Geometry check sheet. Reference: the model listing, model coordinates, mm. A direction names the side the tool comes from. Round coordinates to 2 decimals unless told otherwise and drop trailing zeros. Order: outer loops, then holes, each group sorted by start corner. A loop starts at its lowest first (then second) coordinate and runs counter-clockwise, first axis right, second up.
(1) Cross-section at B-B on x = 0. Enter the section's corners in (y, z).
(2) Draft check along Y on faces 1 (the face through (13, -6, -1)), 2 (the face through (7.483, -6.069, -0.784)), 3 (the face through (9, -15, -1)), 4 (the face through (-9, 15, -1)). Enter one of: pulls with the +Y half, pulls with the -Y half, needs draft (parallel to the pull), parting line crosses it, or undercut.
(3) Set-up check for faces 5 (the face through (-5, -2, -56)), 6 (the face through (6, 13, -1)): record each of +Z, -Z, +X, -X, +Y, -Y from which the full face is reachable in a straight line by a thin tool's end or side.
(4) Cross-section at A-A on y = 11.25. Enter the section's corners in (x, z), and give its area (3 significant figures).
(5) Thickness scan on L1, parallel to Y at x = 10.25, z = -46.5; L2, parallel to Y at x = 0, z = 0.5. Record the ranges inside material, lowest first.
(6) Gauge pin test, flat ends, axial feed: P1, Ø3, axis at y = -3, z = 41.5, coming from the -X side; P2, Ø0.8, axis at x = 4.5, z = 27.5, coming from the -Y side; P3, Ø0.8, axis at x = -4.5, z = -4, coming from the +Y side. Record the tip position at first contact, or that the pin passes through.
Autodesk Inventor part; units mm, degrees
ref_plane "YZ Plane" through (0, 0, 0) normal (1, 0, 0) x (0, 1, 0)
ref_plane "XZ Plane" through (0, 0, 0) normal (0, 1, 0) x (-1, 0, 0)
ref_plane "XY Plane" through (0, 0, 0) normal (0, 0, 1) x (1, 0, 0)
sketch "Sketch1" plane through (0, 0, 0) normal (0, 0, 1) x (1, 0, 0)
  circle A0 centre (0, 0) radius 5
  arc A1 (-13, 15) -> (-15, 13) centre (-13, 13) ccw
  arc A2 (-15, -13) -> (-13, -15) centre (-13, -13) ccw
  arc A3 (13, -15) -> (15, -13) centre (13, -13) ccw
  arc A4 (15, 13) -> (13, 15) centre (13, 13) ccw
  arc A5 (-13, 14) -> (-14, 13) centre (-13, 13) ccw
  arc A6 (-14, -13) -> (-13, -14) centre (-13, -13) ccw
  arc A7 (13, -14) -> (14, -13) centre (13, -13) ccw
  arc A8 (14, 13) -> (13, 14) centre (13, 13) ccw
  line L0 (14, -14) -> (-14, 14) construction
  line L1 (-14, -14) -> (14, 14) construction
  line L2 (15, -15) -> (-15, 15) construction
  line L3 (-15, -15) -> (15, 15) construction
  line L4 (-13, 15) -> (-8, 15)
  line L5 (-8, 13) -> (-8, 8) construction
  line L6 (-9.4142, 8) -> (-13, 8)
  line L7 (-15, 8) -> (-15, 13)
  line L8 (-13, -15) -> (-8, -15)
  line L9 (-8, -13) -> (-8, -9.4142)
  line L10 (-9.4142, -8) -> (-13, -8)
  line L11 (-15, -8) -> (-15, -13)
  line L12 (13, -15) -> (8, -15)
  line L13 (8, -13) -> (8, -9.4142)
  line L14 (9.4142, -8) -> (13, -8)
  line L15 (15, -8) -> (15, -13)
  line L16 (13, 15) -> (8, 15)
  line L17 (8, 13) -> (8, 9.4142)
  line L18 (9.4142, 8) -> (13, 8)
  line L19 (15, 8) -> (15, 13)
  line L20 (-13, 9) -> (-10, 9)
  line L21 (-9, 10) -> (-9, 13)
  line L22 (-10, 14) -> (-13, 14)
  line L23 (-14, 13) -> (-14, 10)
  line L24 (13, 9) -> (10, 9)
  line L25 (9, 10) -> (9, 13)
  line L26 (10, 14) -> (13, 14)
  line L27 (14, 13) -> (14, 10)
  line L28 (13, -9) -> (10, -9)
  line L29 (9, -10) -> (9, -13)
  line L30 (10, -14) -> (13, -14)
  line L31 (14, -13) -> (14, -10)
  line L32 (-13, -9) -> (-10, -9)
  line L33 (-9, -10) -> (-9, -13)
  line L34 (-10, -14) -> (-13, -14)
  line L35 (-14, -13) -> (-14, -10)
  line L36 (-14, 13) -> (-14, 10)
  line L37 (-14, -10) -> (-14, -13)
  line L38 (-14, -13) -> (-14, -10)
  line L39 (-14, 10) -> (-14, 13)
  line L40 (13, -15) -> (5, -15)
  line L41 (-5, -15) -> (-13, -15)
  line L42 (13, -15) -> (5, -15) construction
  line L43 (0, -15) -> (-13, -15) construction
  line L44 (4, -13) -> (8, -13)
  line L45 (-8, -13) -> (-4, -13)
  line L46 (10, -9) -> (13, -9)
  line L47 (14, -10) -> (14, -13)
  line L48 (13, -14) -> (10, -14)
  line L49 (9, -13) -> (9, -10)
  line L50 (5, -14) -> (5, -15)
  line L51 (13, -14) -> (10, -14)
  line L52 (5, -14) -> (4, -14)
  line L53 (4, -14) -> (5, -14)
  line L54 (10, -14) -> (13, -14)
  line L55 (-4, -14) -> (-5, -14)
  line L56 (-10, -14) -> (-13, -14)
  line L57 (-13, -14) -> (-10, -14)
  line L58 (-5, -14) -> (-4, -14)
  line L59 (14, -13) -> (14, -10)
  line L60 (14, 10) -> (14, 13)
  line L61 (14, 13) -> (14, 10)
  line L62 (14, -10) -> (14, -13)
  line L63 (-5, -14) -> (-5, -15)
  line L64 (10, 14) -> (13, 14)
  line L65 (13, 14) -> (10, 14)
  line L66 (-10, 14) -> (-13, 14)
  line L67 (-13, 14) -> (-10, 14)
  line L68 (-5, 15) -> (-5, 14)
  line L69 (-13, 15) -> (-5, 15)
  line L70 (5, 15) -> (13, 15)
  line L71 (-15, 15) -> (-5, 15) construction
  line L72 (5, 15) -> (15, 15) construction
  line L73 (5, 15) -> (5, 14)
  line L74 (8, 13) -> (4, 13)
  line L75 (5, 14) -> (4, 14)
  line L76 (-5, 14) -> (-4, 14)
  line L77 (4, 14) -> (5, 14)
  line L78 (-4, 13) -> (-8, 13)
  line L79 (-4, 14) -> (-5, 14)
  line L80 (4, 13) -> (4, 14)
  line L81 (-4, 13) -> (-4, 14)
  line L82 (-4, -14) -> (-4, -13)
  line L83 (4, -14) -> (4, -13)
  line L84 (-8, 9.4142) -> (-4.1919, 5.6061)
  line L85 (8, 9.4142) -> (4.1919, 5.6061)
  line L86 (9.4142, 8) -> (5.6061, 4.1919)
  line L87 (5.6061, -4.1919) -> (9.4142, -8)
  line L88 (4.1919, -5.6061) -> (8, -9.4142)
  line L89 (-4.1919, -5.6061) -> (-8, -9.4142)
  line L90 (-5.6061, -4.1919) -> (-9.4142, -8)
  line L91 (-9.4142, 8) -> (-5.6061, 4.1919)
  arc A9 (4.1919, 5.6061) -> (-4.1919, 5.6061) centre (0, 0) ccw
  arc A10 (5.6061, -4.1919) -> (5.6061, 4.1919) centre (0, 0) ccw
  arc A11 (-5.6061, 4.1919) -> (-5.6061, -4.1919) centre (0, 0) ccw
  arc A12 (-4.1919, -5.6061) -> (4.1919, -5.6061) centre (0, 0) ccw
  line L92 (-8, 13) -> (-8, 9.4142)
  line L93 (-15, -13) -> (-15, -5) construction
  line L94 (-15, -13) -> (-15, -5)
  line L95 (-15, 5) -> (-15, 13)
  line L96 (15, -5) -> (15, -13) construction
  line L97 (15, 13) -> (15, 5)
  line L98 (15, -5) -> (15, -13)
  line L99 (-14, -4) -> (-14, -5)
  line L100 (14, -4) -> (14, -5)
  line L101 (14, 4) -> (14, 5)
  line L102 (-14, 4) -> (-14, 5)
  line L103 (-13, 8) -> (-13, 4)
  line L104 (13, 4) -> (13, 8)
  line L105 (13, -8) -> (13, -4)
  line L106 (-13, -4) -> (-13, -8)
  line L107 (-14, -5) -> (-15, -5)
  line L108 (15, -5) -> (14, -5)
  line L109 (15, 5) -> (14, 5)
  line L110 (-14, 5) -> (-15, 5)
  line L111 (13, 4) -> (14, 4)
  line L112 (-14, 4) -> (-13, 4)
  line L113 (-14, -4) -> (-13, -4)
  line L114 (13, -4) -> (14, -4)
  arc A13 (-13, -9) -> (-14, -10) centre (-13, -10) ccw
  arc A14 (-9, -10) -> (-10, -9) centre (-10, -10) ccw
  arc A15 (-10, -14) -> (-9, -13) centre (-10, -13) ccw
  arc A16 (10, -9) -> (9, -10) centre (10, -10) ccw
  arc A17 (9, -13) -> (10, -14) centre (10, -13) ccw
  arc A18 (14, -10) -> (13, -9) centre (13, -10) ccw
  arc A19 (10, 14) -> (9, 13) centre (10, 13) ccw
  arc A20 (9, 10) -> (10, 9) centre (10, 10) ccw
  arc A21 (13, 9) -> (14, 10) centre (13, 10) ccw
  arc A22 (-9, 13) -> (-10, 14) centre (-10, 13) ccw
  arc A23 (-10, 9) -> (-9, 10) centre (-10, 10) ccw
  arc A24 (-14, 10) -> (-13, 9) centre (-13, 10) ccw
  point P0 (15, -15)
  point P1 (-5.5858, -7)
  dimension "d0" = 30
  dimension "d1" = 30
  dimension "d2" = 10
  dimension "d4" = 2
  dimension "d11" = 28
  dimension "d12" = 7
  dimension "d13" = 7
  dimension "d15" = 1
  dimension "d16" = 1
  dimension "d17" = 1
  dimension "d18" = 1
  dimension "d19" = 5
  dimension "d23" = 30
  dimension "d27" = 1
  dimension "d30" = 3.5858
  dimension "d31" = 2
  dimension "d32" = 16
  dimension "d33" = 8
  dimension "d34" = 6
  dimension "d35" = 5.5858
extrude "Extrusion1" add sketch "Sketch1" along normal mid plane 112
properties part number "3030T-slot(hor)" material "Aluminum 6061"
Found:
1. outline: (-7, -56) - (-5, -56) - (-5, 56) - (-7, 56) - close; (5, -56) - (7, -56) - (7, 56) - (5, 56) - close
2. face 1: undercut
2. face 2: undercut
2. face 3: pulls with the -Y half
2. face 4: pulls with the +Y half
3. face 5: -Z, +X, -X, +Y, -Y
3. face 6: +Z, -Z
4. outline: (-15, -56) - (-14, -56) - (-14, 56) - (-15, 56) - close; (-9, -56) - (-8, -56) - (-8, 56) - (-9, 56) - close; (8, -56) - (9, -56) - (9, 56) - (8, 56) - close; (14, -56) - (15, -56) - (15, 56) - (14, 56) - close
4. area: 448 mm2
5. L1: y = -15 to -14, -9 to -8, 8 to 9, 14 to 15
5. L2: y = -7 to -5, 5 to 7
6. P1: stops at x = -14
6. P2: stops at y = -14
6. P3: stops at y = 14
